The listing builds one solid part. Answer for the finished solid, in the listing's coordinates (mm). A direction names the side the tool comes from. Coordinates: 2 decimals unless noted, no trailing zeros. Order: outer loops, then holes, each group sorted by start corner. A loop starts at its lowest first (then second) coordinate and runs counter-clockwise, first axis right, second up. Notation, with made-up numbers: (-9.5, 28) -> (21.5, 28) arc R20 cw to (21.5, 51) -> close; hole circle Ø7 at (5.5, -3). An arc over 180 degrees is marked (long way). Return JSON: item names as keys, results as strings.
Autodesk Inventor part; units mm, degrees
ref_plane "YZ Plane" through (0, 0, 0) normal (1, 0, 0) x (0, 1, 0)
ref_plane "XZ Plane" through (0, 0, 0) normal (0, 1, 0) x (-1, 0, 0)
ref_plane "XY Plane" through (0, 0, 0) normal (0, 0, 1) x (1, 0, 0)
sketch "Sketch1" plane through (0, 0, 0) normal (0, 0, 1) x (1, 0, 0)
  point P0 (0, 0)
sketch "Sketch2" plane through (0, 0, 0) normal (0, 0, 1) x (1, 0, 0)
  line L0 (0, 0) -> (279.4, 0)
  line L1 (279.4, 0) -> (279.4, 177.8)
  line L2 (279.4, 177.8) -> (0, 177.8)
  line L3 (0, 177.8) -> (0, 0)
extrude "Extrusion1" add sketch "Sketch2" along normal blind 5
fillet "Fillet1" radius 6 4 edges at (0, 177.8, 2.5) (0, 0, 2.5) (279.4, 0, 2.5) (279.4, 177.8, 2.5)
sketch "Sketch3" plane through (0, 0, 5) normal (0, 0, 1) x (1, 0, 0)
  line L0 (258.2444, 76.2) -> (253.2444, 76.2)
  line L1 (253.2444, 76.2) -> (253.2444, 101.6)
  line L2 (253.2444, 101.6) -> (258.2444, 101.6)
  line L3 (258.2444, 101.6) -> (258.2444, 76.2)
  line L4 (6, 0) -> (273.4, 0)
  point P0 (0, 0)
  dimension "d5" = 5
  dimension "d6" = 25.4
  dimension "d7" = 76.2
extrude "Extrusion2" cut sketch "Sketch3" against normal blind 2
sketch "Sketch4" plane through (0, 0, 5) normal (0, 0, 1) x (1, 0, 0)
  point P0 (0, 0)
sketch "Sketch5" plane through (0, 0, 0) normal (0, 0, -1) x (-1, 0, 0)
  line L0 (-273.4, 177.8) -> (-6, 177.8)
  line L1 (-270.0239, 177.8) -> (-248.6645, 177.8)
  line L2 (-248.6645, 177.8) -> (-248.6645, 172.369)
  line L3 (-248.6645, 172.369) -> (-270.0239, 172.369)
  line L4 (-270.0239, 172.369) -> (-270.0239, 177.8)
  line L5 (-6, 0) -> (-273.4, 0)
  line L6 (-270.0239, 0) -> (-248.6645, 0)
  line L7 (-248.6645, 0) -> (-248.6645, 5.4307)
  line L8 (-248.6645, 5.4307) -> (-270.0239, 5.4307)
  line L9 (-270.0239, 5.4307) -> (-270.0239, 0)
  point P0 (0, 0)
  dimension "d10" = 5.4307
  dimension "d11" = 5.431
extrude "Extrusion3" add sketch "Sketch5" along normal blind 15
sketch "Sketch6" plane through (6, 177.8, 5) normal (0, 1, 0) x (1, 0, 0)
  point P0 (-6, 5)
sketch "Sketch7" plane through (6, 177.8, 5) normal (0, 1, 0) x (1, 0, 0)
  circle A0 centre (253.4743, 12.5024) radius 3
  point P0 (-6, 5)
  dimension "d14" = 6
sketch "Sketch8" plane through (6, 0, 5) normal (0, -1, 0) x (1, 0, 0)
  circle A0 centre (254.3422, -12.325) radius 3
  point P0 (-6, -5)
  dimension "d15" = 6
extrude "Extrusion4" add sketch "Sketch8" along normal blind 25.4
extrude "Extrusion5" add sketch "Sketch7" along normal blind 25.4
sketch "Sketch9" plane through (0, 0, 5) normal (0, 0, 1) x (1, 0, 0)
  line L0 (0, 171.8) -> (0, 6)
  line L1 (0, 139.7) -> (1.4974, 139.7)
  line L2 (1.4974, 139.7) -> (1.4974, 38.1)
  line L3 (1.4974, 38.1) -> (0, 38.1)
  line L4 (0, 38.1) -> (0, 139.7)
  line L5 (6, 0) -> (273.4, 0)
  line L6 (273.4, 177.8) -> (6, 177.8)
  point P0 (0, 0)
  point P1 (0, 38.1)
  dimension "d20" = 38.1
  dimension "d21" = 38.1
extrude "Extrusion6" add sketch "Sketch9" along normal blind 2.5
sketch "Sketch13" plane through (0, 0, 0) normal (0, 0, -1) x (-1, 0, 0)
  circle A0 centre (-25.8349, 40.8578) radius 1
  point P0 (0, 0)
  dimension "d32" = 2
extrude "Extrusion8" add sketch "Sketch13" along normal blind 5
sketch "Sketch14" plane through (0, 0, 0) normal (0, 0, -1) x (-1, 0, 0)
  circle A0 centre (-24.7974, 137) radius 1
  line L0 (-248.6645, 177.8) -> (-6, 177.8)
  line L1 (-1.4974, 139.7) -> (-1.4974, 38.1)
  point P0 (0, 0)
  dimension "d35" = 2
  dimension "d36" = 40.8
  dimension "d37" = 23.3
extrude "Extrusion9" add sketch "Sketch14" along normal blind 5
sketch "Sketch15" plane through (0, 0, 0) normal (0, 0, -1) x (-1, 0, 0)
  point P0 (0, 0)
sketch "Sketch16" plane through (0, 0, 5) normal (0, 0, 1) x (1, 0, 0)
  point P0 (0, 0)
properties part number "base"
1. The part is cut by section C-C on y = 61. Give the vertices of the cut face in (x, z).
Answer block:
{"outline": "(0, 0) -> (279.4, 0) -> (279.4, 5) -> (1.5, 5) -> (1.5, 7.5) -> (0, 7.5) -> close"}
2. The part is cut by section A-A on y = 87. Give the vertices of the cut face in (x, z), and give its area (3 significant figures).
Answer block:
{"outline": "(0, 0) -> (279.4, 0) -> (279.4, 5) -> (258.24, 5) -> (258.24, 3) -> (253.24, 3) -> (253.24, 5) -> (1.5, 5) -> (1.5, 7.5) -> (0, 7.5) -> close", "area": "1,390 mm2"}
3. Consider line 1 (Z direction, x = 79.5, y = 124.5); line 2 (Y direction, x = 224, z = 3.75); line 3 (X direction, y = 61, z = 5.5). Determine where each line is inside the solid, lowest interval first. Write a range as from..to.
Answer block:
{"line 1": "z = 0..5", "line 2": "y = 0..177.8", "line 3": "x = 0..1.5"}
4. Each of these flat-tipped pins is pushed along its axis until it touches: pin 1 Ø1 at (x, z) = (256, 4) entering from +Y; pin 2 Ø1.5 at (x, y) = (256.5, 87) entering from +Z; pin 3 Ø6 at (y, z) = (176, -9) entering from -X. Where does it stop, or does it pass through?
Answer block:
{"pin 1": "stops at y = 177.8", "pin 2": "stops at z = 3", "pin 3": "stops at x = 248.66"}
5. Determine the mould class of faces 1 (the face through (259, 5.431, -7)), 2 (the face through (259, 203.2, -8)), 3 (the face through (259, 172.369, -7)), 4 (the face through (263.113, -12.522, -6.176)) for opening direction Y: pulls with the +Y half, pulls with the -Y half, needs draft (parallel to the pull), parting line crosses it, or undercut.
Answer block:
{"face 1": "undercut", "face 2": "pulls with the +Y half", "face 3": "undercut", "face 4": "needs draft"}
6. The part is cut by section B-B on x = 154.5. Give the vertices of the cut face in (y, z), and give its area (3 significant figures).
Answer block:
{"outline": "(0, 0) -> (177.8, 0) -> (177.8, 5) -> (0, 5) -> close", "area": "889 mm2"}
7. For faces 5 (the face through (259, 175, -15)), 6 (the face through (277.689, 175.996, 2.535)), 7 (the face through (248.664, 175, -7)), 8 (the face through (262.246, 190.322, -8.651)), 9 (the face through (270.024, 175, -7)), determine the directions among +Z, -Z, +X, -X, +Y, -Y from which every point of the face is accessible in a straight line to the end or side of a thin tool.
Answer block:
{"face 5": "-Z, +X, -X, +Y, -Y", "face 6": "+Z, -Z, +X, +Y", "face 7": "-Z, -X, +Y, -Y", "face 8": "+Y", "face 9": "-Z, +X, +Y, -Y"}
8. The part is cut by section D-D on y = 168. Give the vertices of the cut face in (x, z), and give its area (3 significant figures).
Answer block:
{"outline": "(0, 0) -> (279.4, 0) -> (279.4, 5) -> (0, 5) -> close", "area": "1,400 mm2"}
